Geometry check sheet. Reference: the model listing, model coordinates, mm. A direction names the side the tool comes from. Round coordinates to 2 decimals unless told otherwise and drop trailing zeros. Write each loop counter-clockwise with the first axis right and the second up, starting at its lowest first coordinate (ties: lowest second). Pieces come first, ordered by that corner, then holes.
Item 1: Access from +Z, -Z, +X, -X, +Y, -Y to the whole of each face (thin tool, end or side, straight path). Record for faces 1 (the face through (0.62, 1.91, -0.71)), 2 (the face through (0, 3, 2)).
Item 2: Cross-section at D-D (y = 3.6). Enter the section's corners in (x, z).
Item 3: Depth check by flat-ended pin: P1, Ø2.5, axis at y = 3, z = 1, coming from the -X side. Enter the tip coordinate at first touch or a pass-through.
Item 4: Cross-section at B-B (x = 1.85). Enter the section's corners in (y, z), then the cut area to 3 significant figures.
Item 5: Cross-section at C-C (z = 2.55). Enter the section's corners in (x, y) (3 decimals).
Item 6: Scan lines: probe 1 along X at (y, z) = (2.25, 1.65); probe 2 along Y at (x, z) = (1.4, -2.7). Record each from-to range of solid material in increasing order.
Item 7: Cross-section at A-A (y = 2.2). Enter the section's corners in (x, z).
from build123d import *

# Parameters (mm, degrees)
SKETCH1_W           = 6
SKETCH1_H           = 6
BOSS_EXTRUDE1_DEPTH = 5
CUT_EXTRUDE9_DEPTH  = 23.5
CUT_EXTRUDE10_START = -3
CUT_EXTRUDE10_DEPTH = 3


# Read off the part's stored shape, not the designer's step: Cut-Extrude10
with BuildPart() as part:
    # Sketch1 → Boss-Extrude1 (new body)
    with BuildSketch(Plane(origin=(0, 0, 0), x_dir=(1, 0, 0), z_dir=(0, 1, 0))):
        Rectangle(SKETCH1_W, SKETCH1_H)
    extrude(amount=BOSS_EXTRUDE1_DEPTH)

    # Sketch12 → Cut-Extrude9 (cut)
    with BuildSketch(Plane.ZY.offset(3)):
        Polygon((-3, 0), (3, 5), (-3, 5), align=None)
    extrude(amount=-CUT_EXTRUDE9_DEPTH, mode=Mode.SUBTRACT)

    # Cut-Extrude10 outline → Cut-Extrude10 (cut)
    with BuildSketch(Plane.ZY.offset(3).offset(CUT_EXTRUDE10_START)):
        Polygon((3, 5), (0, 2.5), (3, 0), align=None)
    extrude(amount=CUT_EXTRUDE10_DEPTH, mode=Mode.SUBTRACT)


solid = part.part
Resolved:
1. face 1: -Z, +X, -X, +Y
1. face 2: +Z, -X, +Y
2. outline: (0, 1.32) - (3, 1.32) - (3, 3) - (0, 3) - close
3. P1: stops at x = -3
4. outline: (0, -3) - (5, 3) - (0, 3) - close
4. area: 15.0 mm2
5. outline: (-3, 0) - (3, 0) - (3, 4.625) - (0, 4.625) - (0, 0.375) - (-3, 0.375) - close
6. probe 1: x = 0 to 3
6. probe 2: y = 0 to 0.25
7. outline: (-3, -0.36) - (3, -0.36) - (3, 3) - (0, 3) - (0, 0.36) - (-3, 0.36) - close
